```python
from build123d import *

# Parameters (mm, degrees)
BOSS_EXTRUDE1_DEPTH     = 400
CUT_EXTRUDE1_DEPTH      = 401.906229685
CUT_EXTRUDE1_DEPTH_BACK = 401.906229685
SKETCH2_R               = 6
CUT_EXTRUDE2_DEPTH      = 401.906229685
CUT_EXTRUDE2_DEPTH_BACK = 401.906229685
SKETCH3_R               = 3.38


with BuildPart() as part:
    # Sketch1 → Boss-Extrude1 (new body)
    with BuildSketch(Plane.XY):
        with BuildLine():
            Line((-14.05, 19.05), (14.05, 19.05))
            ThreePointArc((14.05, 19.05), (17.585533906, 17.585533906), (19.05, 14.05))
            Line((19.05, 14.05), (19.05, -14.05))
            ThreePointArc((19.05, -14.05), (17.585533906, -17.585533906), (14.05, -19.05))
            Line((14.05, -19.05), (-14.05, -19.05))
            ThreePointArc((-14.05, -19.05), (-17.585533906, -17.585533906), (-19.05, -14.05))
            Line((-19.05, -14.05), (-19.05, 14.05))
            ThreePointArc((-19.05, 14.05), (-17.585533906, 17.585533906), (-14.05, 19.05))
        make_face()
        with BuildLine():
            Line((-15.875, 14.05), (-15.875, -14.05))
            ThreePointArc((-15.875, -14.05), (-15.340469876, -15.340469876), (-14.05, -15.875))
            Line((-14.05, -15.875), (14.05, -15.875))
            ThreePointArc((14.05, -15.875), (15.340469876, -15.340469876), (15.875, -14.05))
            Line((15.875, -14.05), (15.875, 14.05))
            ThreePointArc((15.875, 14.05), (15.340469876, 15.340469876), (14.05, 15.875))
            Line((14.05, 15.875), (-14.05, 15.875))
            ThreePointArc((-14.05, 15.875), (-15.340469876, 15.340469876), (-15.875, 14.05))
        make_face(mode=Mode.SUBTRACT)
    extrude(amount=BOSS_EXTRUDE1_DEPTH)

    # Sketch2 → Cut-Extrude1 (cut, two sides: drawn at the far end of the back side and taken through both)
    with BuildSketch(Plane(origin=(0, 0, 0), x_dir=(0, 0, -1), z_dir=(1, 0, 0)).offset(-CUT_EXTRUDE1_DEPTH_BACK)):
        with Locations((-375, 0)):
            Circle(SKETCH2_R)
        with Locations((-25, 0)):
            Circle(SKETCH2_R)
    extrude(amount=CUT_EXTRUDE1_DEPTH + CUT_EXTRUDE1_DEPTH_BACK, mode=Mode.SUBTRACT)

    # Sketch3 → Cut-Extrude2 (cut, two sides: drawn at the far end of the back side and taken through both)
    with BuildSketch(Plane(origin=(0, 0, 0), x_dir=(1, 0, 0), z_dir=(0, 1, 0)).offset(-CUT_EXTRUDE2_DEPTH_BACK)):
        with Locations(Location((0, -325, 0), (0, 0, 90))):
            Circle(SKETCH3_R)
        with Locations(Location((0, -75, 0), (0, 0, 90))):
            Circle(SKETCH3_R)
    extrude(amount=CUT_EXTRUDE2_DEPTH + CUT_EXTRUDE2_DEPTH_BACK, mode=Mode.SUBTRACT)


solid = part.part
```
Could you check a few things on this model? Use its own coordinates, in mm. A direction names the side the tool comes from. Round coordinates to 2 decimals unless told otherwise and drop trailing zeros. Write each loop counter-clockwise with the first axis right and the second up, starting at its lowest first coordinate (ties: lowest second). Pieces come first, ordered by that corner, then holes. Notation, with made-up numbers: M 60.5,46 L 76.5,46 A17 cw 76.5,54 Z; hole C 19,-12.75 d6. An arc over 180 degrees is marked long. Answer in a Markdown table with one row per item. Add a question column.
Q1. If we mould it in two halves opening along Y, with no side actions, what happens to faces 3 (the cylindrical face through (-17.485, 1.802, 369.277)), 4 (the flat face through (0, -19.05, 197)), 5 (the flat face through (-15.875, 0, 197)), 6 (the cylindrical face through (-0.149, -17.485, 78.377))? For each: +Y half, -Y half, draft (parallel to the pull), parting line (faces both ways), or undercut.
Q2. Imagine slicing it at A-A (y = -10.5). Please give me the cut outline in (x, z) (3 decimals).
Q3. Will this pin go through, and if not, where does the flat tip stop? pin 1 Ø5.5 at (x, z) = (0, 75) entering from -Y.
Q4. Imagine slicing it at C-C (z = 75). Please give me the cut outline in (x, y) (3 decimals), then the cut area to 3 significant figures.
Q5. If I drill on line 1 (Z direction, x = -16, y = 0); line 2 (Y direction, x = 13, z = 310) (3 decimals), over which ranges is the centre line in solid material (lowest first)? Write a range as from..to.
Q6. Imagine slicing it at B-B (x = 0). Please give me the cut outline in (y, z) (3 decimals), then the cut area to 3 significant figures.
Q7. Imagine slicing it at D-D (z = 231.5). Please give me the cut outline in (x, y) (3 decimals).
Q8. On a 3-axis mill with a long thin cutter (end or side, diameter ignored), from which of +Z, -Z, +X, -X, +Y, -Y can I reach the whole of each face in a straight line? I mean faces 1 (the flat face through (15.875, 0, 197)), 2 (the cylindrical face through (-0.149, 17.44, 78.377)). Say none if no direction works.
Values:
| question | item | result |
|---|---|---|
| 1 | face 3 | undercut |
| 1 | face 4 | -Y half |
| 1 | face 5 | undercut |
| 1 | face 6 | draft |
| 2 | outline | M -19.05,0 L -15.875,0 L -15.875,400 L -19.05,400 Z; M 15.875,0 L 19.05,0 L 19.05,400 L 15.875,400 Z |
| 3 | pin 1 | through |
| 4 | outline | M -19.05,-14.05 A5 ccw -14.05,-19.05 L -3.38,-19.05 L -3.38,-15.875 L -14.05,-15.875 A1.825 cw -15.875,-14.05 L -15.875,14.05 A1.825 cw -14.05,15.875 L -3.38,15.875 L -3.38,19.05 L -14.05,19.05 A5 ccw -19.05,14.05 Z; M 3.38,-19.05 L 14.05,-19.05 A5 ccw 19.05,-14.05 L 19.05,14.05 A5 ccw 14.05,19.05 L 3.38,19.05 L 3.38,15.875 L 14.05,15.875 A1.825 cw 15.875,14.05 L 15.875,-14.05 A1.825 cw 14.05,-15.875 L 3.38,-15.875 Z |
| 4 | area | 382 mm^2 |
| 5 | line 1 | 0..19, 31..369, 381..400 |
| 5 | line 2 | -19.05..-15.875, 15.875..19.05 |
| 6 | outline | M -19.05,0 L -15.875,0 L -15.875,71.62 L -19.05,71.62 Z; M -19.05,78.38 L -15.875,78.38 L -15.875,321.62 L -19.05,321.62 Z; M -19.05,328.38 L -15.875,328.38 L -15.875,400 L -19.05,400 Z; M 15.875,0 L 19.05,0 L 19.05,71.62 L 15.875,71.62 Z; M 15.875,78.38 L 19.05,78.38 L 19.05,321.62 L 15.875,321.62 Z; M 15.875,328.38 L 19.05,328.38 L 19.05,400 L 15.875,400 Z |
| 6 | area | 2,450 mm^2 |
| 7 | outline | M -19.05,-14.05 A5 ccw -14.05,-19.05 L 14.05,-19.05 A5 ccw 19.05,-14.05 L 19.05,14.05 A5 ccw 14.05,19.05 L -14.05,19.05 A5 ccw -19.05,14.05 Z; hole M -15.875,-14.05 A1.825 ccw -14.05,-15.875 L 14.05,-15.875 A1.825 ccw 15.875,-14.05 L 15.875,14.05 A1.825 ccw 14.05,15.875 L -14.05,15.875 A1.825 ccw -15.875,14.05 Z |
| 8 | face 1 | +Z, -Z |
| 8 | face 2 | +Y, -Y |
